Part model, mm, in its own coordinate system. Coordinates: 2 decimals unless noted, no trailing zeros. Order: outer loops, then holes, each group sorted by start corner. A loop starts at its lowest first (then second) coordinate and runs counter-clockwise, first axis right, second up.
1) Cut at C-C (y = -67). List the corners of the cut face in (x, z) (3 decimals), and give its area (3 significant figures).
2) Wall check: L1, parallel to Y at x = 185.5, z = 0.85 (3 decimals); L2, parallel to Y at x = -6, z = 2.65; L3, parallel to X at y = 8.5, z = 0.95 (3 decimals). Give the ranges that are in metal, low to high.
3) Cut at B-B (z = 0.8). Give the number of separate pieces and of enclosed holes in the cut face, and give its area (3 significant figures).
4) Pin check, flat tips, straight feed: pin 1 Ø1 at (y, z) = (-50, 1) entering from +X; pin 2 Ø1 at (x, z) = (120, 1.5) entering from -Y; pin 3 Ø1.5 at (y, z) = (-73, 2.5) entering from +X. Stop position of each tip, or through.
5) Cut at A-A (x = 181). List the corners of the cut face in (y, z) (3 decimals).
```python
from build123d import *

# Parameters (mm, degrees)
SKETCH1_R           = 129.2733
SKETCH1_R_2         = 116.5733
BOSS_EXTRUDE1_DEPTH = 3.175
SKETCH2_W           = 3.175
SKETCH2_H           = 8.466666666
CUT_EXTRUDE1_DEPTH  = 3.175
CUT_EXTRUDE6_START  = -3.175
CUT_EXTRUDE6_DEPTH  = 3.175
SKETCH4_W           = 25.4
SKETCH4_H           = 3.175
CUT_EXTRUDE7_DEPTH  = 3.175


with BuildPart() as part:
    # Sketch1 → Boss-Extrude1 (new body)
    # profile 1 of 3: a face of its own
    with BuildSketch(Plane.XY):
        with BuildLine():
            Line((-206.375, -12.7), (-128.647954095, -12.7))
            ThreePointArc((-128.647954095, -12.7), (-129.2733, 0), (-128.647954095, 12.7))
            Line((-128.647954095, 12.7), (-206.375, 12.7))
            Line((-206.375, 12.7), (-206.375, -12.7))
        make_face()
    # profile 2 of 3: a face of its own
    with BuildSketch(Plane.XY):
        Circle(SKETCH1_R)
        Circle(SKETCH1_R_2, mode=Mode.SUBTRACT)
    # profile 3 of 3: a face of its own
    with BuildSketch(Plane.XY):
        with BuildLine():
            ThreePointArc((129.2733, 0), (129.116868877, -6.357693322), (128.647954095, -12.7))
            Line((128.647954095, -12.7), (206.375, -12.7))
            Line((206.375, -12.7), (206.375, 12.7))
            Line((206.375, 12.7), (128.647954095, 12.7))
            ThreePointArc((128.647954095, 12.7), (129.116868877, 6.357693322), (129.2733, 0))
        make_face()
    extrude(amount=BOSS_EXTRUDE1_DEPTH)

    # Sketch2 → Cut-Extrude1 (cut)
    with BuildSketch(Plane.XY.offset(3.175)):
        with Locations((-204.7875, 0)):
            Rectangle(SKETCH2_W, SKETCH2_H)
    cut_extrude1 = extrude(amount=-CUT_EXTRUDE1_DEPTH, mode=Mode.SUBTRACT)

    # Mirror1: Cut-Extrude1 across plane
    add(cut_extrude1.mirror(Plane(origin=(0, 0, 0), x_dir=(0, 0, 1), z_dir=(1, 0, 0))), mode=Mode.SUBTRACT)

    # Sketch3 → Cut-Extrude6 (cut)
    with BuildSketch(Plane.XY.offset(3.175).offset(CUT_EXTRUDE6_START)):
        with BuildLine():
            Line((-116.400222392, -6.35), (-129.100222392, -6.35))
            Line((-129.100222392, -6.35), (-129.100222392, 6.35))
            Line((-129.100222392, 6.35), (-116.400222392, 6.35))
            ThreePointArc((-116.400222392, 6.35), (-116.5733, 0), (-116.400222392, -6.35))
        make_face()
    cut_extrude6 = extrude(amount=CUT_EXTRUDE6_DEPTH, mode=Mode.SUBTRACT)

    # Mirror2: Cut-Extrude6 across plane
    add(cut_extrude6.mirror(Plane(origin=(0, 0, 0), x_dir=(0, 0, 1), z_dir=(1, 0, 0))), mode=Mode.SUBTRACT)

    # Sketch4 → Cut-Extrude7 (cut)
    with BuildSketch(Plane.XY.offset(3.175)):
        with Locations((187.325, -4.7625)):
            Rectangle(SKETCH4_W, SKETCH4_H)
    cut_extrude7 = extrude(amount=-CUT_EXTRUDE7_DEPTH, mode=Mode.SUBTRACT)

    # Mirror3: Cut-Extrude7 across plane
    add(cut_extrude7.mirror(Plane(origin=(0, 0, 0), x_dir=(0, 0, 1), z_dir=(1, 0, 0))), mode=Mode.SUBTRACT)


solid = part.part
```
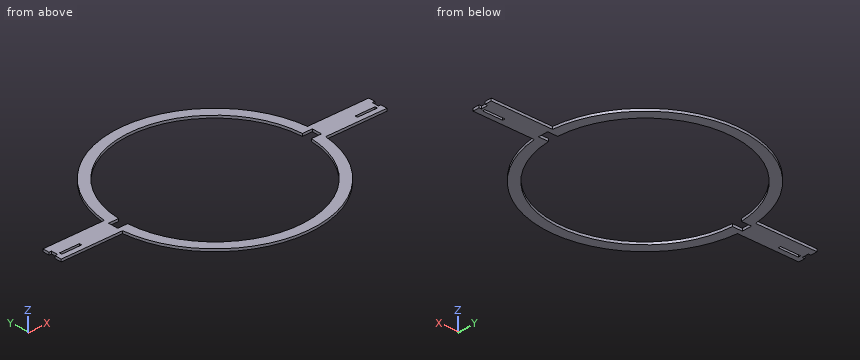
Geometry check:
1. outline: (-110.556, 0) - (-95.396, 0) - (-95.396, 3.175) - (-110.556, 3.175) - close; (95.396, 0) - (110.556, 0) - (110.556, 3.175) - (95.396, 3.175) - close
1. area: 96.3 mm2
2. L1: y = -12.7 to -6.35, -3.175 to 12.7
2. L2: y = -129.13 to -116.42, 116.42 to 129.13
2. L3: x = -206.375 to -116.263, 116.263 to 206.375
3. separate pieces: 1
3. enclosed holes: 3
3. area: 13,200 mm2
4. pin 1: stops at x = 119.42
4. pin 2: stops at y = -49.31
4. pin 3: stops at x = 107.2
5. outline: (-12.7, 0) - (-6.35, 0) - (-6.35, 3.175) - (-12.7, 3.175) - close; (-3.175, 0) - (12.7, 0) - (12.7, 3.175) - (-3.175, 3.175) - close
